```python
from build123d import *

# Parameters (mm, degrees)
F0_W      = 15.2
F0_H      = 19.2
F1_DEPTH  = 1.6
F2_R      = 6
F3_DEPTH  = 7.2
F3_TAPER  = -3
F4_R      = 1.25
F5_DEPTH  = 3.5
F6_R      = 1
F7_DEPTH  = 25
F8_W      = 7.5
F8_H      = 2.5
F9_DEPTH  = 2.5
F11_W     = 0.6
F11_H     = 0.6
F12_DEPTH = 7.3
F13_W     = 0.6
F13_H     = 0.6
F14_DEPTH = 7.5


with BuildPart() as f1:
    # F0 (on Top) → F1 (new body)
    with BuildSketch(Plane.XY):
        Rectangle(F0_W, F0_H)
    extrude(amount=F1_DEPTH)

    # F2 (on face) → F3 (join)
    with BuildSketch(Plane.XY.offset(1.6)):
        with Locations((0, 0.6)):
            Circle(F2_R)
    extrude(amount=F3_DEPTH, taper=F3_TAPER)

    # F4 (on face) → F5 (cut)
    with BuildSketch(Plane.XY.offset(8.8)):
        with Locations((0, 0.6)):
            Circle(F4_R)
    extrude(amount=-F5_DEPTH, mode=Mode.SUBTRACT)

    # F6 (on face) → F7 (cut)
    with BuildSketch(Plane.XY.offset(1.6)):
        with Locations((-5.1, 7.1)):
            Circle(F6_R)
        with Locations((5.1, 7.1)):
            Circle(F6_R)
    extrude(amount=-F7_DEPTH, mode=Mode.SUBTRACT)

    # F8 (on face) → F9 (join)
    with BuildSketch(Plane.XY.offset(1.6)):
        with Locations((0, -7.85)):
            Rectangle(F8_W, F8_H)
    extrude(amount=F9_DEPTH)

    # F11 (on offset) → F12 (join)
    with BuildSketch(Plane.XY.offset(-1.5)):
        with Locations((0, -7.85)):
            Rectangle(F11_W, F11_H)
        with Locations((2.4999999441, -7.85)):
            Rectangle(F11_W, F11_H)
        with Locations((-2.4999999441, -7.85)):
            Rectangle(F11_W, F11_H)
        with Locations((0, 3.95)):
            Rectangle(F11_W, F11_H)
        with Locations((0, -2.45)):
            Rectangle(F11_W, F11_H)
    extrude(amount=F12_DEPTH)

    # F13 (on face) → F14 (join)
    with BuildSketch(Plane(origin=(0, -7.55, 0), x_dir=(-1, 0, 0), z_dir=(0, 1, 0))):
        with Locations((2.4999999441, 5.5)):
            Rectangle(F13_W, F13_H)
        Polygon((0.3, 5.8), (0, 5.8), (-0.3, 5.8), (-0.3, 5.2), (0, 5.2), (0.3, 5.2), align=None)
        with Locations((-2.4999999441, 5.5)):
            Rectangle(F13_W, F13_H)
    extrude(amount=-F14_DEPTH)


solid = f1.part
```
The model under review builds one solid part; all positions refer to its coordinate system, in mm. A direction names the side the tool comes from. Round coordinates to 2 decimals unless told otherwise and drop trailing zeros. Order: outer loops, then holes, each group sorted by start corner. A loop starts at its lowest first (then second) coordinate and runs counter-clockwise, first axis right, second up. Notation, with made-up numbers: M 80.5,-18.5 L 94.5,-18.5 A12 ccw 94.5,-5.5 Z; hole C 50,77 d4. An arc over 180 degrees is marked long. Use a Markdown table: item, result.
1) Consider section C-C (z = 7). Write out the cut boundary in (x, y).
Report:
| item | result |
|---|---|
| outline | C 0,0.6 d12.57; hole C 0,0.6 d2.5 |
2) Tool access review of faces 4 (the face through (-2.8, -10.5, 5.5)), 5 (the face through (0.3, -10.5, 5.5)), 6 (the face through (0, 1, 5.3)): name each direction out of +Z, -Z, +X, -X, +Y, -Y from which nothing blocks a thin tool from reaching the whole face with its end or side.
Report:
| item | result |
|---|---|
| face 4 | +Z, -X, -Y |
| face 5 | +Z, -Y |
| face 6 | +Z |
3) Draft analysis for pull direction Y (two halves, no side actions). For faces 1 (the face through (-0.27, -0.62, 7.07)), 2 (the face through (0, 9.6, 1)), 3 (the face through (0, -1, 8.8)), state which applies: released by +Y, released by -Y, zero draft, split by the parting line, or undercut.
Report:
| item | result |
|---|---|
| face 1 | undercut |
| face 2 | released by +Y |
| face 3 | zero draft |
4) Consider section A-A (z = 3.5). Write out the cut boundary in (x, y).
Report:
| item | result |
|---|---|
| outline | C 0,0.6 d12.2; M -3.75,-9.1 L 3.75,-9.1 L 3.75,-6.6 L -3.75,-6.6 Z |
5) Consider section B-B (y = 7.5). Write out the cut boundary in (x, z).
Report:
| item | result |
|---|---|
| outline | M -7.6,0 L -6.02,0 L -6.02,1.6 L -7.6,1.6 Z; M -4.18,0 L 4.18,0 L 4.18,1.6 L -4.18,1.6 Z; M 6.02,0 L 7.6,0 L 7.6,1.6 L 6.02,1.6 Z |
6) Wall thickness on line 1 along Y through (x, z) = (-5.1, 0.5); line 2 along Y through (x, z) = (0, 6.5); line 3 along X through (y, z) = (-0.5, 8.5): over which ranges is each line inside the solid? List them lowest first. Write a range as [from, to].
Report:
| item | result |
|---|---|
| line 1 | [-9.6, 6.1], [8.1, 9.6] |
| line 2 | [-5.66, -0.65], [1.85, 6.86] |
| line 3 | [-6.27, -0.59], [0.59, 6.27] |
7) Insertion check: pin 1 (4 mm diameter, centred on y = 5.5, z = 6.5, fed in from +X); pin 2 (0.7 mm diameter, centred on y = -8, z = -0.5, fed in from -X); pin 3 (1.9 mm diameter, centred on y = -10.5, z = 4.5, fed in from +X). Each pin has a flat end and moves straight along its axis. Give the tip position at first contact, or say it passes through.
Report:
| item | result |
|---|---|
| pin 1 | x = 5.55 |
| pin 2 | x = -2.8 |
| pin 3 | x = 2.8 |
